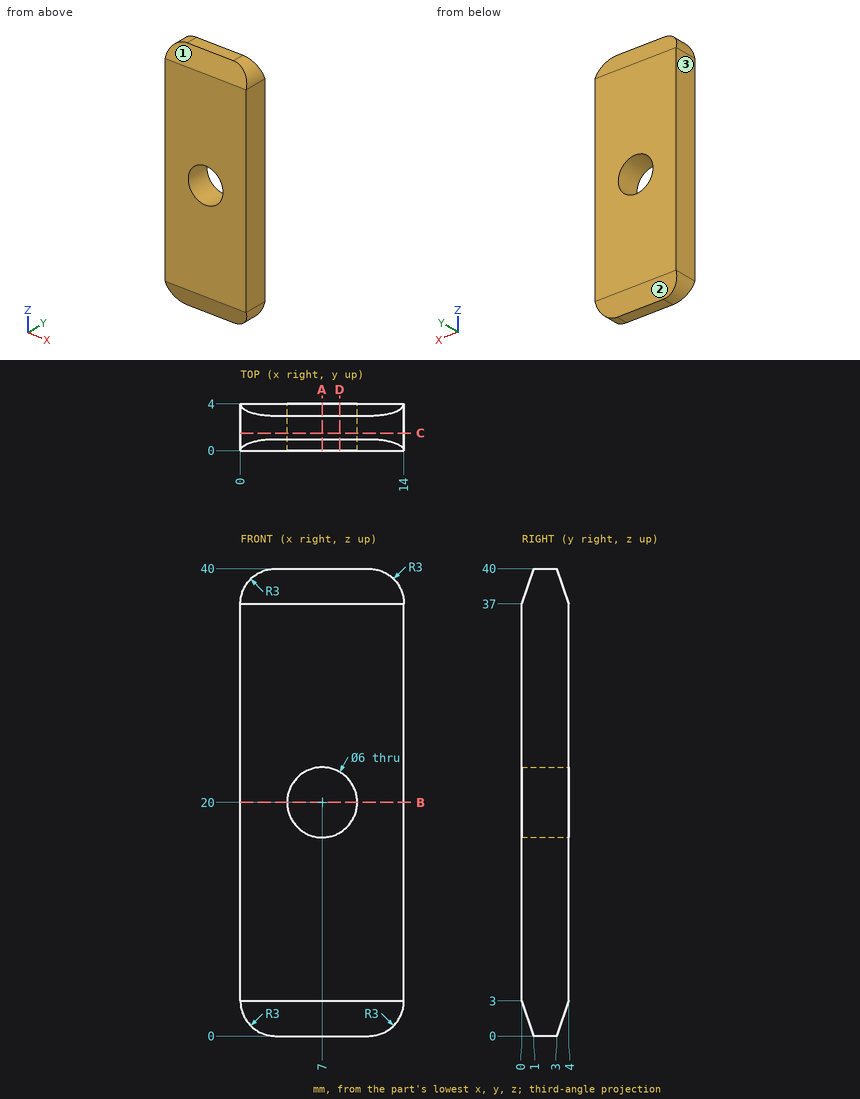
Geometry: see drawing. Coordinates: mm, zero at the bounding-box minimum. Give positions to 0.01 mm unless a question says otherwise; leave off trailing zeros. Loops run counter-clockwise (first coordinate to the right, second up) from the corner with the lowest first, then second, coordinate; pieces in that order, holes last. Notation, with made-up numbers: (43.5, 61.25) - (75.5, 61.25) arc R18 ccw to (75.5, 96.25) - close; hole circle Ø8 at (63.5, 35.5). An arc over 180 degrees is marked (long way). Use CSV: the item, a comma, the result in double quotes. Start each with the question number.
1. Section C-C (y = 1.5). Output: boundary loops of the cut face in (x, z).
2. Section B-B (z = 20). Output: boundary loops of the cut face in (x, y).
3. Ray query, L1, parallel to Z at x = 7, y = 2.4; L2, parallel to X at y = 3.55, z = 17.5; L3, parallel to Z at x = 2, y = 2.25. Return the intervals inside material, ascending.
4. Section A-A (x = 7). Output: boundary loops of the cut face in (y, z).
5. Pin query (flat end, axial travel): pin 1 (1.5 mm diameter, centred on x = 2, y = 0.5, fed in from -Z). Return the tip coordinate at first contact, or that it passes through.
6. Section D-D (x = 8.5). Output: boundary loops of the cut face in (y, z), then the cut area to 3 significant figures.
7. Draft query along Y for the marked faces 1, 2 and 3. Return one class per face: +Y half, -Y half, draft (parallel to the pull), parting line (faces both ways), or undercut.
Response:
1,outline,"(0, 3) arc R3 ccw to (3, 0) - (11, 0) arc R3 ccw to (14, 3) - (14, 37) arc R3 ccw to (11, 40) - (3, 40) arc R3 ccw to (0, 37) - close; hole circle Ø6 at (7, 20)"
2,outline,"(0, 0) - (4, 0) - (4, 4) - (0, 4) - close; (10, 0) - (14, 0) - (14, 4) - (10, 4) - close"
3,L1,"0 to 17, 23 to 40"
3,L2,"0 to 5.34, 8.66 to 14"
3,L3,"0.17 to 39.83"
4,outline,"(0, 3) - (1, 0) - (3, 0) - (4, 3) - (4, 17) - (0, 17) - close; (0, 23) - (4, 23) - (4, 37) - (3, 40) - (1, 40) - (0, 37) - close"
5,pin 1,"z = 0.03"
6,outline,"(0, 3) - (1, 0) - (3, 0) - (4, 3) - (4, 17.4) - (0, 17.4) - close; (0, 22.6) - (4, 22.6) - (4, 37) - (3, 40) - (1, 40) - (0, 37) - close"
6,area,"133 mm²"
7,face 1,"-Y half"
7,face 2,"+Y half"
7,face 3,"draft"
